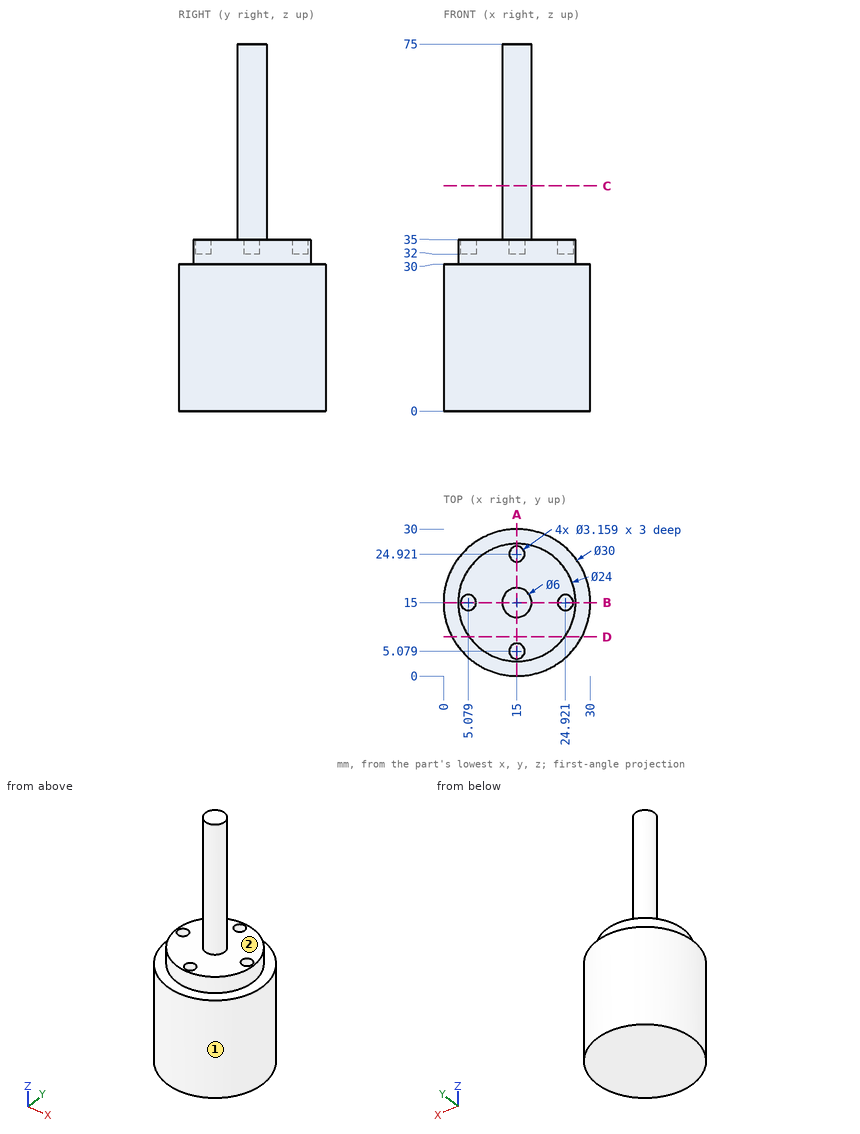
The figure shows three views and two pictorial views of one solid part (mm, origin at its lowest corner). Answer the questions. A direction names the side the tool comes from. Give positions to 0.01 mm unless a question says otherwise; leave off trailing zeros. Order: outer loops, then holes, each group sorted by start corner. A loop starts at its lowest first (then second) coordinate and runs counter-clockwise, first axis right, second up. Notation, with made-up numbers: M 71.25,36 L 85.25,36 A21 ccw 85.25,74 Z; hole C 55.25,30 d3. An arc over 180 degrees is marked long. Return JSON: item names as keys, results as strings.
1) Section A-A, the plane x = 15 is taken. Write down the section's boundary in (y, z), plus the area to 3 significant figures.
Resolved:
{"outline": "M 0,0 L 30,0 L 30,30 L 27,30 L 27,35 L 26.5,35 L 26.5,32 L 23.34,32 L 23.34,35 L 18,35 L 18,75 L 12,75 L 12,35 L 6.66,35 L 6.66,32 L 3.5,32 L 3.5,35 L 3,35 L 3,30 L 0,30 Z", "area": "1,240 mm^2"}
2) Straight lines are drawn through the part: line 1 along Y through (x, z) = (15, 33.6); line 2 along Z through (x, y) = (8, 7.25); line 3 along Z through (x, y) = (24.25, 23.25). For each, find the intervals that lie inside material, in ascending order. Write a range as [from, to].
Resolved:
{"line 1": "[3, 3.5], [6.66, 23.34], [26.5, 27]", "line 2": "[0, 35]", "line 3": "[0, 30]"}
3) Each of these flat-tipped pins is pushed along its axis until it touches: pin 1 (12 mm diameter, centred on x = 3, z = 10.5, fed in from +Y); pin 2 (1 mm diameter, centred on x = 25.5, y = 5.5, fed in from +Z); pin 3 (3.5 mm diameter, centred on x = 14.5, y = 25.5, fed in from +Z). Where does it stop, or does it pass through?
Resolved:
{"pin 1": "y = 28.75", "pin 2": "z = 30", "pin 3": "z = 35"}
4) Section D-D, the plane y = 8 is taken. Write down the section's boundary in (x, z).
Resolved:
{"outline": "M 1.73,0 L 28.27,0 L 28.27,30 L 24.75,30 L 24.75,35 L 5.25,35 L 5.25,30 L 1.73,30 Z"}
5) Section C-C, the plane z = 46 is taken. Write down the section's boundary in (x, y), plus the area to 3 significant figures.
Resolved:
{"outline": "C 15,15 d6", "area": "28.3 mm^2"}
6) A tool of negligible diameter and unlimited length cuts with its end or side. For the marked faces 1 and 2, from which of +Z, -Z, +X, -X, +Y, -Y can it reach the whole face along a straight path? Write none if from no direction.
Resolved:
{"face 1": "+Z, -Z", "face 2": "+Z"}
